CAD build for the part. Positions are in the model's coordinates, mm. Round coordinates to 2 decimals unless told otherwise and drop trailing zeros. Order: outer loops, then holes, each group sorted by start corner. A loop starts at its lowest first (then second) coordinate and runs counter-clockwise, first axis right, second up. Notation, with made-up numbers: (29, 9) -> (63, 9) arc R15 cw to (63, 38) -> close; hole circle Ø6 at (30.25, -36). An arc over 180 degrees is marked (long way). Return JSON: item names as keys, results as strings. Group by question number.
Q1. Cut at B-B (y = 78). Write the cut outline in (x, z) (1 decimal), then the cut area to 3 significant figures.
Q2. Cut at A-A (z = 11). Write the cut outline in (x, y) (1 decimal), then the cut area to 3 significant figures.
Q3. Probe line 1 along X through (y, z) = (82.5, 9); line 2 along Y through (x, z) = (-175.5, 10); line 3 along X through (y, z) = (96, 6.25). List the from-to ranges inside material, lowest first.
Q4. Flat gauge pins, fed straight in: pin 1 (1 mm diameter, centred on y = 33.5, z = 9.5, fed in from -X); pin 2 (6 mm diameter, centred on x = -2.5, z = 9.5, fed in from -Y); pin 3 (8 mm diameter, centred on y = 36, z = 6, fed in from -X). Where does each tip first touch, or does it go through?
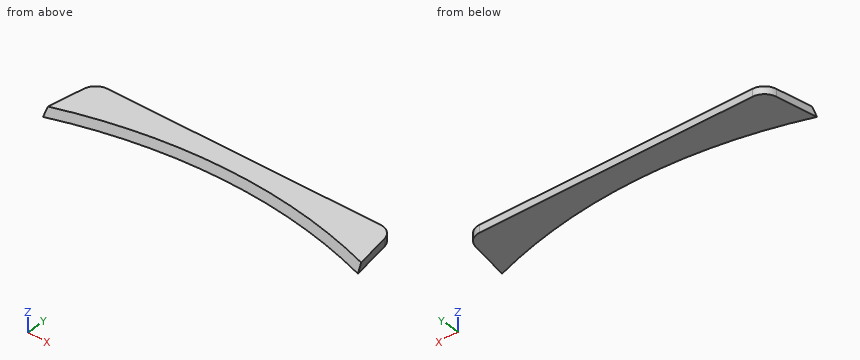
from build123d import *

# Parameters (mm, degrees)
F1_DEPTH = 15.875
F2_SIZE2 = 9.165426
F2_SIZE  = 15.87499


# Not quite as in the source:
# - a fillet or chamfer is up to 0.001 mm smaller than in the source, because OpenCascade refuses the exact size


with BuildPart() as f1:
    # F0 (on Top) → F1 (new body)
    with BuildSketch(Plane.XY):
        with BuildLine():
            ThreePointArc((-333.375, 0), (0, 56.2515384878), (333.375, 0))
            Line((333.375, 0), (318.4555045755, 84.6126631589))
            ThreePointArc((318.4555045755, 84.6126631589), (308.1393220024, 102.4808155156), (288.7512407253, 109.5375))
            Line((288.7512407253, 109.5375), (-288.7512407253, 109.5375))
            ThreePointArc((-288.7512407253, 109.5375), (-308.1393220024, 102.4808155156), (-318.4555045755, 84.6126631589))
            Line((-318.4555045755, 84.6126631589), (-333.375, 0))
        make_face()
    extrude(amount=F1_DEPTH)

    # F2 (size 15.875 and 9.1654355234 in the source; OpenCascade refuses exactly that, so slightly less here)
    f2_edges = [f1.edges().sort_by_distance(p)[0] for p in [
        (0, 56.251538, 15.875),
    ]]
    f2_side = f1.faces().sort_by_distance((0, 56.251538, 7.9375))[0]
    chamfer(f2_edges, length=F2_SIZE, length2=F2_SIZE2, reference=f2_side)


solid = f1.part
Solution:
{
 "1": {"outline": "(-319.6, 0) -> (319.6, 0) -> (319.6, 15.9) -> (-319.6, 15.9) -> close", "area": "10,100 mm²"},
 "2": {"outline": "(-332.1, 7.2) arc R1022.4 cw to (332.1, 7.2) -> (318.5, 84.6) arc R30.2 ccw to (288.8, 109.5) -> (-288.8, 109.5) arc R30.2 ccw to (-318.5, 84.6) -> close", "area": "41,200 mm²"},
 "3": {"line 1": "x = -318.83 to 318.83", "line 2": "y = 46.84 to 109.54", "line 3": "x = -313.92 to 313.92"},
 "4": {"pin 1": "stops at x = -327.56", "pin 2": "stops at y = 60", "pin 3": "stops at x = -327.73"}
}
